```python
from build123d import *

# Parameters (mm, degrees)
F0_R     = 1.25
F1_DEPTH = 12
F2_R     = 11
F2_R_2   = 1.25
F3_DEPTH = 8
F4_R     = 2


with BuildPart() as f1:
    # F0 (on Front) → F1 (new body)
    with BuildSketch(Plane.XZ):
        with BuildLine():
            Line((5.8942117522, 24.8663670726), (17.3253891795, 21.2155887136))
            ThreePointArc((17.3253891795, 21.2155887136), (19.3737008087, 20.0819692322), (20.832276605, 18.2507864708))
            Line((20.832276605, 18.2507864708), (14.5059308294, 30.5141249497))
            Line((14.5059308294, 30.5141249497), (-15.0105899225, 39.9408245069))
            Line((-15.0105899225, 39.9408245069), (-17.4444421618, 32.3200395554))
            Line((-17.4444421618, 32.3200395554), (5.8942117522, 24.8663670726))
        make_face()
        with BuildLine():
            Line((5.8942117522, 24.8663670726), (9.7844112864, 17.3253891795))
            ThreePointArc((9.7844112864, 17.3253891795), (12.7492135292, 20.832276605), (17.3253891795, 21.2155887136))
            Line((17.3253891795, 21.2155887136), (5.8942117522, 24.8663670726))
        make_face()
        with BuildLine():
            ThreePointArc((17.3253891795, 21.2155887136), (12.7492135292, 20.832276605), (9.7844112864, 17.3253891795))
            ThreePointArc((9.7844112864, 17.3253891795), (9.5715291903, 16.4237065871), (9.5, 15.5))
            ThreePointArc((9.5, 15.5), (14.5762934129, 9.5715291903), (21.2155887136, 13.6746108205))
            ThreePointArc((21.2155887136, 13.6746108205), (21.4284708097, 14.5762934129), (21.5, 15.5))
            ThreePointArc((21.5, 15.5), (21.3306800474, 16.9153339482), (20.832276605, 18.2507864708))
            ThreePointArc((20.832276605, 18.2507864708), (19.3737008087, 20.0819692322), (17.3253891795, 21.2155887136))
        make_face()
        with BuildLine():
            ThreePointArc((17.15, 15.5), (15.5, 13.85), (13.85, 15.5))
            ThreePointArc((13.85, 15.5), (15.5, 17.15), (17.15, 15.5))
        make_face(mode=Mode.SUBTRACT)
        with BuildLine():
            ThreePointArc((4.7370094053, 1.5211576496), (10.2697554893, 4.9403923414), (14.5, 0))
            ThreePointArc((14.5, 0), (14.0831583376, -1.9986644672), (12.9021361391, -3.6640782867))
            Line((12.9021361391, -3.6640782867), (16.8483243992, 0))
            Line((16.8483243992, 0), (21.2155887136, 13.6746108205))
            ThreePointArc((21.2155887136, 13.6746108205), (14.5762934129, 9.5715291903), (9.5, 15.5))
            Line((9.5, 15.5), (9.2014362293, 15.5))
            Line((9.2014362293, 15.5), (4.7370094053, 1.5211576496))
        make_face()
        with BuildLine():
            ThreePointArc((12.9021361391, -3.6640782867), (14.0831583376, -1.9986644672), (14.5, 0))
            ThreePointArc((14.5, 0), (10.2697554893, 4.9403923414), (4.7370094053, 1.5211576496))
            ThreePointArc((4.7370094053, 1.5211576496), (6.819580417, -4.2208234811), (12.9021361391, -3.6640782867))
        make_face()
        with Locations((9.5, 0)):
            Circle(F0_R, mode=Mode.SUBTRACT)
        with BuildLine():
            Line((9.7844112864, 17.3253891795), (9.2014362293, 15.5))
            Line((9.2014362293, 15.5), (9.5, 15.5))
            ThreePointArc((9.5, 15.5), (9.5715291903, 16.4237065871), (9.7844112864, 17.3253891795))
        make_face()
    extrude(amount=F1_DEPTH)

    # F2 (on face) → F3 (cut)
    with BuildSketch(Plane.XZ.offset(12)):
        with Locations((9.5, 0)):
            Circle(F2_R)
        with Locations((9.5, 0)):
            Circle(F2_R_2, mode=Mode.SUBTRACT)
    extrude(amount=-F3_DEPTH, mode=Mode.SUBTRACT)

    # F4
    f4_edges = [f1.edges().sort_by_distance(p)[0] for p in [
        (-17.444442, -6, 32.32004),
        (5.894212, -6, 24.866367),
        (9.784411, -6, 17.325389),
        (7.717857, -8, 10.854675),
        (18.749677, -8, 5.953442),
        (14.505931, -6, 30.514125),
    ]]
    fillet(f4_edges, radius=F4_R)


solid = f1.part
```
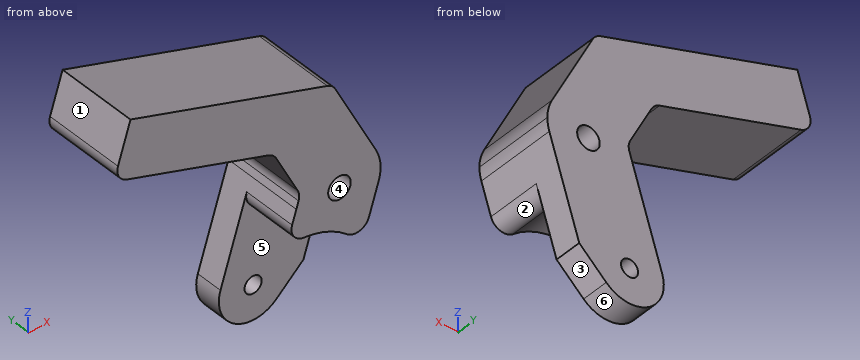
The listing builds one solid part. Answer for the finished solid, in the listing's coordinates (mm). Face numbers are marked on the shaded views. A direction names the side the tool comes from. Give positions to 0.01 mm unless a question says otherwise; leave off trailing zeros. Order: outer loops, then holes, each group sorted by start corner. A loop starts at its lowest first (then second) coordinate and runs counter-clockwise, first axis right, second up. Notation, with made-up numbers: (-33.75, 31) -> (7.25, 31) arc R36 cw to (7.25, 65) -> close; hole circle Ø6 at (-35.75, 73). An arc over 180 degrees is marked (long way). Write each question's results on one line, items separated by ' | '.
Q1. The part is cut by section A-A, the plane x = 15.5. Give the vertices of the cut face in (y, z).
Checked values:
outline: (-12, 9.22) -> (-4, 9.22) -> (-4, -1.25) -> (0, -1.25) -> (0, 13.85) -> (-12, 13.85) -> close; (-12, 17.15) -> (0, 17.15) -> (0, 28.59) -> (-12, 28.59) -> close
Q2. Each of these flat-tipped pins is pushed along its axis until it touches: P1, Ø6, axis at x = 17, z = 3.5, coming from the -Y side; P2, Ø2, axis at y = -6.5, z = 35.5, coming from the -X side; P3, Ø1, axis at x = 12.5, y = -1.5, coming from the -Z side. Where does it stop, or does it pass through?
Checked values:
P1: stops at y = -4 | P2: stops at x = -16.75 | P3: stops at z = -4.33
Q3. Determine the mould class of the marked faces 3, 4, 5 and 6 for opening direction X: pulls with the +X half, pulls with the -X half, needs draft (parallel to the pull), parting line crosses it, or undercut.
Checked values:
face 3: pulls with the +X half | face 4: undercut | face 5: needs draft | face 6: parting line crosses it
Q4. The part is cut by section D-D, the plane x = 3.5. Give the vertices of the cut face in (y, z).
Checked values:
outline: (-12, 25.63) -> (0, 25.63) -> (0, 34.03) -> (-12, 34.03) -> close
Q5. Straight lines are drawn through the part: probe 1 along Y at (x, z) = (19, 7); probe 2 along Z at (x, y) = (15.5, -3.5); probe 3 along Z at (x, y) = (-9.5, -4.75). For each, find the intervals that lie inside material, in ascending order. Write a range as from..to.
Checked values:
probe 1: y = -4..0 | probe 2: z = -1.25..13.85, 17.15..28.59 | probe 3: z = 29.78..38.18
Q6. The part is cut by section B-B, the plane y = -5.5. Give the vertices of the cut face in (x, z), and give its area (3 significant figures).
Checked values:
outline: (-16.84, 34.23) arc R2 ccw to (-15.54, 31.71) -> (5.11, 25.12) arc R2 cw to (6.27, 24.13) -> (9.4, 18.06) arc R2 cw to (9.53, 16.54) -> (8.59, 13.57) arc R2 ccw to (10.34, 10.97) arc R11 cw to (16.62, 8.39) arc R2 ccw to (19.82, 9.3) -> (21.22, 13.67) arc R6 ccw to (20.83, 18.25) -> (14.89, 29.78) arc R2 ccw to (13.72, 30.77) -> (-15.01, 39.94) -> close; hole circle Ø3.3 at (15.5, 15.5) | area: 424 mm^2
Q7. Which of the six approach directions +Z, -Z, +X, -X, +Y, -Y give full straight-line access (tool end or side, diameter ignored) to the marked faces 1 and 2?
Checked values:
face 1: +Z, -X, +Y, -Y | face 2: -Z, -Y
Q8. The part is cut by section C-C, the plane z = 33. Give the vertices of the cut face in (x, y).
Checked values:
outline: (-16.83, -12) -> (6.72, -12) -> (6.72, 0) -> (-16.83, 0) -> close
